Check sheet for the drawn part. Datum: minimum x, y, z corner. Units: mm. A direction names the side the tool comes from. Give positions to 0.01 mm unless a question says otherwise; leave off trailing zeros. Loops run counter-clockwise (first coordinate to the right, second up) from the corner with the lowest first, then second, coordinate; pieces in that order, holes last. Notation, with made-up numbers: M 68.5,36 L 85.5,36 A12 ccw 85.5,44 Z; hole C 29.25,0.5 d3. An arc over 180 degrees is marked long. Write each question's results on one line, items separated by ' | '. Start each with the question number.
1. Sectioned sample at C-C on z = 1.45. Record the cut outline in (x, y), and give its area (3 significant figures).
2. Sectioned sample at A-A on y = 21. Record the cut outline in (x, z), and give its area (3 significant figures).
3. Go/stop test with flat-tipped pins: pin 1 (1 mm diameter, centred on x = 18, z = 1, fed in from +Y); pin 2 (1.6 mm diameter, centred on x = 35, z = 3, fed in from -Y); pin 3 (1 mm diameter, centred on y = 30, z = 3.5, fed in from -X); pin 4 (21 mm diameter, centred on x = 23, y = 13.5, fed in from -Z). Record where each tip stops, or that it passes through.
4. Material ranges on line 1 along Y through (x, z) = (22.5, 1.2); line 2 along X through (y, z) = (13, 3.55); line 3 along Y through (x, z) = (39, 3.75), recorded low to high.
5. Tool access check on the marked faces 1 and 2. Record the directions out of +Z, -Z, +X, -X, +Y, -Y that give a thin tool (end or side, any length) a straight path to the whole face; none if there is none.
6. Sectioned sample at B-B on x = 22.5. Record the cut outline in (y, z), and give its area (3 significant figures).
7. Sectioned sample at D-D on x = 36. Record the cut outline in (y, z), and give its area (3 significant figures).
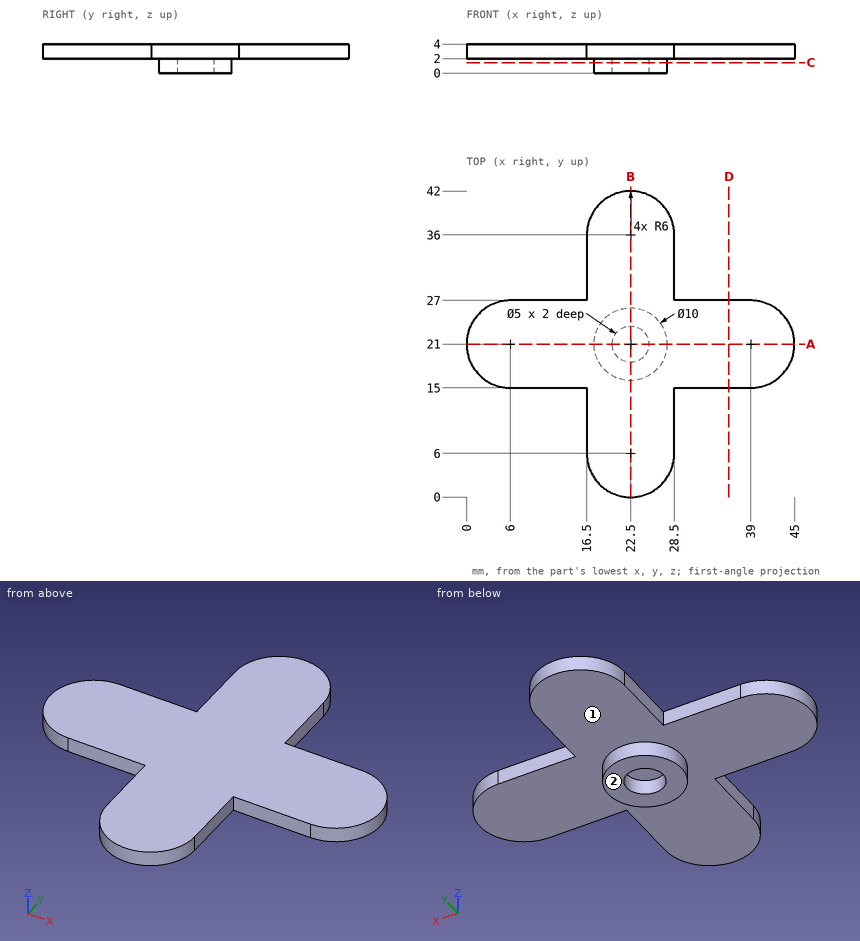
Output values:
1) outline: C 22.5,21 d10; hole C 22.5,21 d5 | area: 58.9 mm2
2) outline: M 0,2 L 17.5,2 L 17.5,0 L 20,0 L 20,2 L 25,2 L 25,0 L 27.5,0 L 27.5,2 L 45,2 L 45,4 L 0,4 Z | area: 100 mm2
3) pin 1: y = 24 | pin 2: y = 15 | pin 3: x = 16.5 | pin 4: z = 0
4) line 1: 16 to 18.5, 23.5 to 26 | line 2: 16.5 to 28.5 | line 3: 15 to 27
5) face 1: -Z | face 2: -Z, +X, -X, +Y, -Y
6) outline: M 0,2 L 16,2 L 16,0 L 18.5,0 L 18.5,2 L 23.5,2 L 23.5,0 L 26,0 L 26,2 L 42,2 L 42,4 L 0,4 Z | area: 94.0 mm2
7) outline: M 15,2 L 27,2 L 27,4 L 15,4 Z | area: 24.0 mm2
